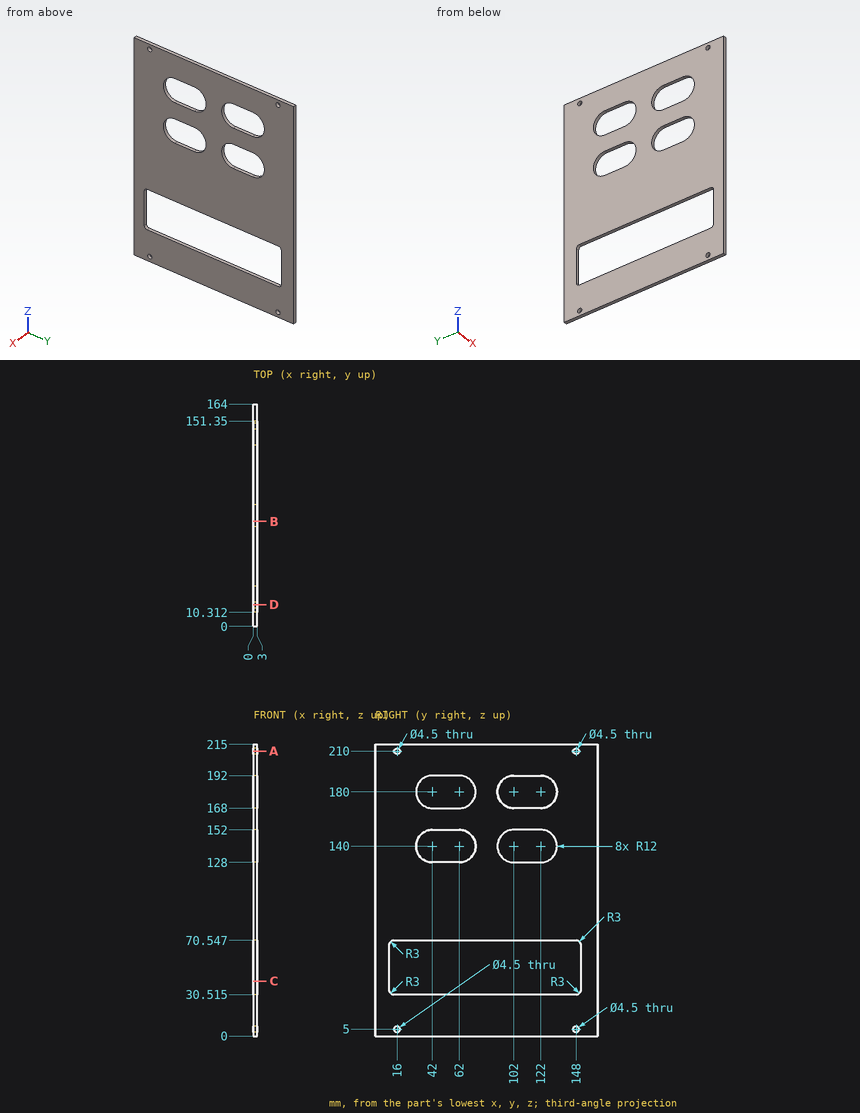
Verification items for this drawing (mm, ordinates from the low corner). Give positions to 0.01 mm unless a question says otherwise; leave off trailing zeros. Write each loop counter-clockwise with the first axis right and the second up, starting at its lowest first coordinate (ties: lowest second). Pieces come first, ordered by that corner, then holes. Notation, with made-up numbers: (45.5, 14) -> (84.5, 14) arc R15 cw to (84.5, 31) -> close; hole circle Ø2 at (75.5, 78.25). An arc over 180 degrees is marked (long way). Use one line per item in the form item = value.
Item 1: Depth check by flat-ended pin: pin 1 Ø10 at (y, z) = (62.5, 189) entering from +X. Enter the tip coordinate at first touch or a pass-through.
Results list:
pin_1 = 3
Item 2: Sectioned sample at B-B on y = 77.5. Enter the section's corners in (x, z) (1 decimal).
Results list:
outline = (0, 0) -> (3, 0) -> (3, 30.5) -> (0, 30.5) -> close; (0, 70.5) -> (3, 70.5) -> (3, 215) -> (0, 215) -> close
Item 3: Sectioned sample at A-A on z = 210. Enter the section's corners in (x, y).
Results list:
outline = (0, 0) -> (3, 0) -> (3, 13.75) -> (0, 13.75) -> close; (0, 18.25) -> (3, 18.25) -> (3, 145.75) -> (0, 145.75) -> close; (0, 150.25) -> (3, 150.25) -> (3, 164) -> (0, 164) -> close
Item 4: Sectioned sample at D-D on y = 16. Count the separate pieces of the cut face and the enclosed holes in it, plus the area to 3 significant figures.
Results list:
separate_pieces = 4
enclosed_holes = 0
area = 498 mm2
Item 5: Scan lines: line 1 (Y direction, x = 1.5, z = 210); line 2 (Y direction, x = 0.4, z = 139); line 3 (Z direction, x = 2.85, y = 44) (1 decimal). Record each from-to range of solid material in increasing order.
Results list:
line_1 = 0 to 13.75, 18.25 to 145.75, 150.25 to 164
line_2 = 0 to 30.04, 73.96 to 90.04, 133.96 to 164
line_3 = 0 to 30.5, 70.5 to 128, 152 to 168, 192 to 215
Item 6: Sectioned sample at C-C on z = 40.5. Enter the section's corners in (x, y).
Results list:
outline = (0, 0) -> (3, 0) -> (3, 10.31) -> (0, 10.31) -> close; (0, 151.35) -> (3, 151.35) -> (3, 164) -> (0, 164) -> close
